Verification items for the finished model (mm, model axes). Face numbers are marked on the shaded views. A direction names the side the tool comes from. Give positions to 0.01 mm unless a question says otherwise; leave off trailing zeros. Write each loop counter-clockwise with the first axis right and the second up, starting at its lowest first coordinate (ties: lowest second). Pieces come first, ordered by that corner, then holes. Notation, with made-up numbers: (-13.5, 41.25) -> (40.5, 41.25) arc R30 cw to (40.5, 78.25) -> close; hole circle Ø2 at (-14, -32). An arc over 180 degrees is marked (long way). Use one line per item in the form item = value. Start each with the question number.
(1) Release check for a two-part mould opening along Y. For the marked faces 4, 5 and 6 record: pulls with the +Y half, pulls with the -Y half, needs draft (parallel to the pull), parting line crosses it, or undercut.
(2) Set-up check for the marked faces 1, 2 and 3: record each of +Z, -Z, +X, -X, +Y, -Y from which the full face is reachable in a straight line by a thin tool's end or side.
(3) Scan lines: L1, parallel to X at y = 9, z = 12.75; L2, parallel to Y at x = -13, z = 3.25; L3, parallel to X at y = 0, z = 18.75. Record each from-to range of solid material in increasing order.
(4) Section check D-D, the plane z = 1.75. State how many separate pieces and enclosed holes the cut face has, plus the area to 3 significant figures.
(5) Section check C-C, the plane x = -12.5. Record the cut outline in (y, z), plus the area to 3 significant figures.
(6) Section check B-B, the plane z = 10. Record the cut outline in (x, y).
(7) Section check A-A, the plane x = 0. Record the cut outline in (y, z), plus the area to 3 significant figures.
(8) Depth check by flat-ended pin: pin 1 Ø1.3 at (x, y) = (-14.5, 0) entering from +Z; pin 2 Ø1.5 at (y, z) = (4, 8) entering from +X. Enter the tip coordinate at first touch or a pass-through.
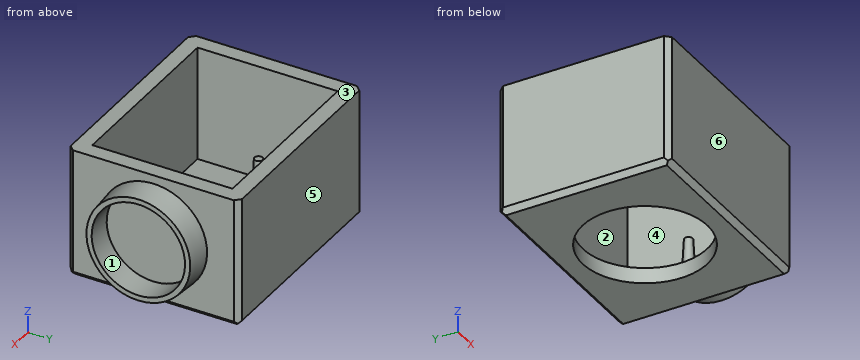
from build123d import *

# Parameters (mm, degrees)
SKETCH_1_W          = 41
SKETCH_1_H          = 33
SKETCH_1_W_2        = 35
SKETCH_1_H_2        = 27
EXTRUDE_1_DEPTH     = 22
SKETCH_6_W          = 41
SKETCH_6_H          = 33
EXTRUDE_1_2_DEPTH   = 3
SKETCH_7_R          = 12
CUT_EXTRUDE_1_DEPTH = 5
CHAMFER_1_SIZE      = 1
CHAMFER_2_SIZE      = 1
CHAMFER_3_SIZE      = 1
CHAMFER_4_SIZE      = 1
SKETCH_8_R          = 1.1
EXTRUDE_3_DEPTH     = 6
EXTRUDE_3_TAPER     = 3
CHAMFER_5_SIZE      = 1
CHAMFER_6_SIZE      = 1
CHAMFER_7_SIZE      = 1
CHAMFER_8_SIZE      = 1
SKETCH_9_R          = 10.35
EXTRUDE_4_DEPTH     = 5
EXTRUDE_4_TAPER     = 4
SKETCH_10_R         = 9
CUT_EXTRUDE_2_DEPTH = 5


with BuildPart() as part:
    # Эскиз1 → Extrude 1 (new body)
    with BuildSketch(Plane.XY):
        Rectangle(SKETCH_1_W, SKETCH_1_H)
        Rectangle(SKETCH_1_W_2, SKETCH_1_H_2, mode=Mode.SUBTRACT)
    extrude(amount=EXTRUDE_1_DEPTH)

    # Эскиз6 → Extrude 1 2 (add)
    with BuildSketch(Plane(origin=(0, 0, 0), x_dir=(-1, 0, 0), z_dir=(0, 0, -1))):
        Rectangle(SKETCH_6_W, SKETCH_6_H)
    extrude(amount=EXTRUDE_1_2_DEPTH)

    # Эскиз7 → Вырез-Вытянуть1 (cut)
    with BuildSketch(Plane(origin=(0, 0, -3), x_dir=(-1, 0, 0), z_dir=(0, 0, -1))):
        Circle(SKETCH_7_R)
    extrude(amount=-CUT_EXTRUDE_1_DEPTH, mode=Mode.SUBTRACT)

    # Фаска1
    chamfer_1_edges = [part.edges().sort_by_distance(p)[0] for p in [
        (0, 16.5, -3),
    ]]
    chamfer(chamfer_1_edges, length=CHAMFER_1_SIZE)

    # Фаска2
    chamfer_2_edges = [part.edges().sort_by_distance(p)[0] for p in [
        (20.5, -0.5, -3),
    ]]
    chamfer(chamfer_2_edges, length=CHAMFER_2_SIZE)

    # Фаска3
    chamfer_3_edges = [part.edges().sort_by_distance(p)[0] for p in [
        (-20.5, -0.5, -3),
    ]]
    chamfer(chamfer_3_edges, length=CHAMFER_3_SIZE)

    # Фаска4
    chamfer_4_edges = [part.edges().sort_by_distance(p)[0] for p in [
        (0, -16.5, -3),
    ]]
    chamfer(chamfer_4_edges, length=CHAMFER_4_SIZE)

    # Эскиз8 → Бобышка-Вытянуть3 (add)
    with BuildSketch(Plane.XY):
        with Locations((14.5, 0)):
            Circle(SKETCH_8_R)
        with Locations((-14.5, 0)):
            Circle(SKETCH_8_R)
    extrude(amount=EXTRUDE_3_DEPTH, taper=EXTRUDE_3_TAPER)

    # Фаска5
    chamfer_5_edges = [part.edges().sort_by_distance(p)[0] for p in [
        (-20.5, 16.5, 10),
    ]]
    chamfer(chamfer_5_edges, length=CHAMFER_5_SIZE)

    # Фаска6
    chamfer_6_edges = [part.edges().sort_by_distance(p)[0] for p in [
        (20.5, 16.5, 10),
    ]]
    chamfer(chamfer_6_edges, length=CHAMFER_6_SIZE)

    # Фаска7
    chamfer_7_edges = [part.edges().sort_by_distance(p)[0] for p in [
        (20.5, -16.5, 10),
    ]]
    chamfer(chamfer_7_edges, length=CHAMFER_7_SIZE)

    # Фаска8
    chamfer_8_edges = [part.edges().sort_by_distance(p)[0] for p in [
        (-20.5, -16.5, 10),
    ]]
    chamfer(chamfer_8_edges, length=CHAMFER_8_SIZE)

    # Эскиз9 → Бобышка-Вытянуть4 (add)
    with BuildSketch(Plane(origin=(20.5, 0, 0), x_dir=(0, 0, -1), z_dir=(1, 0, 0))):
        with Locations((-10, 0)):
            Circle(SKETCH_9_R)
    extrude(amount=EXTRUDE_4_DEPTH, taper=EXTRUDE_4_TAPER)

    # Эскиз10 → Вырез-Вытянуть2 (cut)
    with BuildSketch(Plane(origin=(25.5, 0, 0), x_dir=(0, 0, -1), z_dir=(1, 0, 0))):
        with Locations((-10, 0)):
            Circle(SKETCH_10_R)
    extrude(amount=-CUT_EXTRUDE_2_DEPTH, mode=Mode.SUBTRACT)


solid = part.part
Completed:
q1.face_4 = undercut
q1.face_5 = pulls with the +Y half
q1.face_6 = pulls with the -Y half
q2.face_1 = +X
q2.face_2 = +Z
q2.face_3 = +Z, +X, -X, +Y, -Y
q3.L1 = -20.5 to -17.5, 17.5 to 25.5
q3.L2 = -16.5 to -13.5, 13.5 to 16.5
q3.L3 = -20.5 to -17.5, 17.5 to 20.5
q4.separate_pieces = 3
q4.enclosed_holes = 1
q4.area = 436 mm²
q5.outline = (-16.5, -2) -> (-15.5, -3) -> (15.5, -3) -> (16.5, -2) -> (16.5, 22) -> (13.5, 22) -> (13.5, 0) -> (-13.5, 0) -> (-13.5, 22) -> (-16.5, 22) -> close
q5.area = 230 mm²
q6.outline = (-20.5, -15.5) -> (-19.5, -16.5) -> (19.5, -16.5) -> (20.5, -15.5) -> (20.5, -10.35) -> (25.5, -10) -> (25.5, -9) -> (20.5, -9) -> (20.5, 9) -> (25.5, 9) -> (25.5, 10) -> (20.5, 10.35) -> (20.5, 15.5) -> (19.5, 16.5) -> (-19.5, 16.5) -> (-20.5, 15.5) -> close; hole (-17.5, -13.5) -> (17.5, -13.5) -> (17.5, 13.5) -> (-17.5, 13.5) -> close
q7.outline = (-16.5, -2) -> (-15.5, -3) -> (-12, -3) -> (-12, 0) -> (-13.5, 0) -> (-13.5, 22) -> (-16.5, 22) -> close; (12, -3) -> (15.5, -3) -> (16.5, -2) -> (16.5, 22) -> (13.5, 22) -> (13.5, 0) -> (12, 0) -> close
q7.area = 158 mm²
q8.pin_1 = 6
q8.pin_2 = 20.5
